```python
from build123d import *

# Parameters (mm, degrees)
BOSS_EXTRU_1_DEPTH      = 25
BOSS_EXTRU_2_DEPTH      = 3
ESQUISSE5_W             = 6
ESQUISSE5_H             = 10.8
ESQUISSE5_W_2           = 7
ESQUISSE5_H_2           = 14
ENL_V_MAT_EXTRU_1_DEPTH = 13
ESQUISSE6_R             = 1.7
ENL_V_MAT_EXTRU_2_DEPTH = 13


with BuildPart() as part:
    # Esquisse1 → Boss.-Extru.1 (new body)
    with BuildSketch(Plane.XY):
        with BuildLine():
            Line((-54.225217391, 16.453664596), (0.774782609, 16.453664596))
            ThreePointArc((0.774782609, 16.453664596), (7.845850421, 13.524732408), (10.774782609, 6.453664596))
            Line((10.774782609, 6.453664596), (7.774782609, 6.453664596))
            ThreePointArc((7.774782609, 6.453664596), (5.724530077, 11.403412065), (0.774782609, 13.453664596))
            Line((0.774782609, 13.453664596), (-54.225217391, 13.453664596))
            ThreePointArc((-54.225217391, 13.453664596), (-59.17496486, 11.403412065), (-61.225217391, 6.453664596))
            Line((-61.225217391, 6.453664596), (-64.225217391, 6.453664596))
            ThreePointArc((-64.225217391, 6.453664596), (-61.296285203, 13.524732408), (-54.225217391, 16.453664596))
        make_face()
    extrude(amount=BOSS_EXTRU_1_DEPTH)

    # Esquisse3 → Boss.-Extru.2 (add)
    with BuildSketch(Plane.XY):
        with BuildLine():
            Line((-61.062614557, 7.953664596), (7.612179774, 7.953664596))
            ThreePointArc((7.612179774, 7.953664596), (5.162264802, 11.908020654), (0.774782609, 13.453664596))
            Line((0.774782609, 13.453664596), (-54.225217391, 13.453664596))
            ThreePointArc((-54.225217391, 13.453664596), (-58.612699585, 11.908020654), (-61.062614557, 7.953664596))
        make_face()
    extrude(amount=BOSS_EXTRU_2_DEPTH)

    # Esquisse5 → Enlèv. mat.-Extru.1 (cut)
    with BuildSketch(Plane(origin=(0, 16.453664596, 0), x_dir=(1, 0, 0), z_dir=(0, 1, 0))):
        with Locations((-46.725217391, -12.5)):
            Rectangle(ESQUISSE5_W, ESQUISSE5_H)
        with Locations((-6.725217391, -12.5)):
            Rectangle(ESQUISSE5_W, ESQUISSE5_H)
        with Locations((-26.725217391, -12.5)):
            Rectangle(ESQUISSE5_W_2, ESQUISSE5_H_2)
    extrude(amount=-ENL_V_MAT_EXTRU_1_DEPTH, mode=Mode.SUBTRACT)

    # Esquisse6 → Enlèv. mat.-Extru.2 (cut)
    with BuildSketch(Plane(origin=(0, 0, 0), x_dir=(-1, 0, 0), z_dir=(0, 0, -1))):
        with Locations((-0.774782609, 10.703664596)):
            Circle(ESQUISSE6_R)
        with Locations((26.725217391, 10.703664596)):
            Circle(ESQUISSE6_R)
        with Locations((54.225217391, 10.703664596)):
            Circle(ESQUISSE6_R)
    extrude(amount=-ENL_V_MAT_EXTRU_2_DEPTH, mode=Mode.SUBTRACT)


solid = part.part
```
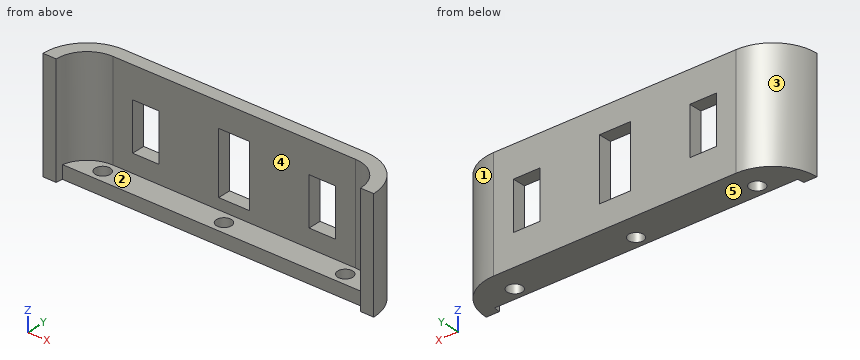
Design review of the part built by this model. Coordinates are the model's own, in mm. Face numbers are marked on the shaded views. A direction names the side the tool comes from. Coordinates: 2 decimals unless noted, no trailing zeros. Write each loop counter-clockwise with the first axis right and the second up, starting at its lowest first coordinate (ties: lowest second). Pieces come first, ordered by that corner, then holes.
1) Machinability: for the marked faces 1 and 2, which of the approach directions +Z, -Z, +X, -X, +Y, -Y give a long, thin tool a straight path to every point of the face, cutting with its end or side? Answer none if there is none.
2) Add section A-A (x = -48). Write out the cut boundary in (y, z), plus the area to 3 significant figures.
3) Add section C-C (z = 4.75). Write out the cut boundary in (x, y), plus the area to 3 significant figures.
4) Add section B-B (z = 16.25). Write out the cut boundary in (x, y).
5) Mouldability with a two-part tool opening along X and no side actions: class the marked faces 3, 4 and 5 as +X half, -X half, draft (parallel to the pull), parting line (faces both ways), or undercut.
6) Insertion check: pin 1 (2.5 mm diameter, centred on x = -31.5, z = 1.5, fed in from -Y); pin 2 (2 mm diameter, centred on x = -51.5, z = 12.5, fed in from -Y); pin 3 (4.5 mm diameter, centred on x = -54.23, y = 10.7, fed in from +Z). Each pin has a flat end and moves straight along its axis. Give the tip position at first contact, or say it passes through.
7) Add section D-D (y = 11.5). Write out the cut boundary in (x, z), plus the area to 3 significant figures.
8) To check wall thickness, follow L1, parallel to X at y = 11, z = 1.5; L2, parallel to X at y = 10, z = 1.5; L3, parallel to Z at x = -11.5, y = 11.5. State the ranges of each line that lie inside material, in increasing order.
Check result:
1. face 1: +Z, -Z, +X, +Y
1. face 2: +Z, -Y
2. outline: (7.95, 0) - (16.45, 0) - (16.45, 7.1) - (13.45, 7.1) - (13.45, 3) - (7.95, 3) - close; (13.45, 17.9) - (16.45, 17.9) - (16.45, 25) - (13.45, 25) - close
2. area: 59.1 mm2
3. outline: (-64.23, 6.45) - (-61.23, 6.45) arc R7 cw to (-54.23, 13.45) - (0.77, 13.45) arc R7 cw to (7.77, 6.45) - (10.77, 6.45) arc R10 ccw to (0.77, 16.45) - (-54.23, 16.45) arc R10 ccw to start
3. area: 245 mm2
4. outline: (-64.23, 6.45) - (-61.23, 6.45) arc R7 cw to (-54.23, 13.45) - (-49.73, 13.45) - (-49.73, 16.45) - (-54.23, 16.45) arc R10 ccw to start; (-43.73, 13.45) - (-30.23, 13.45) - (-30.23, 16.45) - (-43.73, 16.45) - close; (-23.23, 13.45) - (-9.73, 13.45) - (-9.73, 16.45) - (-23.23, 16.45) - close; (-3.73, 13.45) - (0.77, 13.45) arc R7 cw to (7.77, 6.45) - (10.77, 6.45) arc R10 ccw to (0.77, 16.45) - (-3.73, 16.45) - close
5. face 3: -X half
5. face 4: undercut
5. face 5: draft
6. pin 1: stops at y = 7.95
6. pin 2: stops at y = 13.45
6. pin 3: stops at z = 3
7. outline: (-62.86, 0) - (-55.73, 0) - (-55.73, 3) - (-59.08, 3) - (-59.08, 25) - (-62.86, 25) - close; (-52.72, 0) - (-28.23, 0) - (-28.23, 3) - (-52.72, 3) - close; (-25.22, 0) - (-0.73, 0) - (-0.73, 3) - (-25.22, 3) - close; (2.28, 0) - (9.41, 0) - (9.41, 25) - (5.63, 25) - (5.63, 3) - (2.28, 3) - close
7. area: 356 mm2
8. L1: x = -63.13 to -55.9, -52.55 to -28.4, -25.05 to -0.9, 2.45 to 9.68
8. L2: x = -63.58 to -55.77, -52.68 to -28.27, -25.18 to -0.77, 2.32 to 10.12
8. L3: z = 0 to 3
